Verification items for the finished model (mm, model axes). A direction names the side the tool comes from. Coordinates: 2 decimals unless noted, no trailing zeros. Write each loop counter-clockwise with the first axis right and the second up, starting at its lowest first coordinate (ties: lowest second). Pieces come first, ordered by that corner, then holes. Notation, with made-up numbers: (29.5, -21.5) -> (34.5, -21.5) arc R21 ccw to (34.5, 12.5) -> close; hole circle Ø11 at (24, -29). An arc over 180 degrees is marked (long way). Write each question's results on one line, items separated by ' | '. Start each with the question number.
from build123d import *

# Parameters (mm, degrees)
SKETCH1_R                = 21.082
SKETCH1_R_2              = 17.526
BOSS_EXTRUDE1_DEPTH      = 196.85
BOSS_EXTRUDE1_DEPTH_BACK = 196.85
SKETCH2_R                = 3.175
CUT_EXTRUDE1_DEPTH       = 22.082


with BuildPart() as part:
    # Sketch1 → Boss-Extrude1 (new body, two sides)
    with BuildSketch(Plane(origin=(0, 0, 0), x_dir=(0, 0, -1), z_dir=(1, 0, 0))) as boss_extrude1_sk:
        Circle(SKETCH1_R)
        Circle(SKETCH1_R_2, mode=Mode.SUBTRACT)
    extrude(amount=BOSS_EXTRUDE1_DEPTH)
    extrude(boss_extrude1_sk.sketch, amount=-BOSS_EXTRUDE1_DEPTH_BACK)

    # Sketch2 → Cut-Extrude1 (cut, through all)
    with BuildSketch(Plane.XY):
        with Locations((-114.3, 0)):
            Circle(SKETCH2_R)
        with Locations((-165.1, 0)):
            Circle(SKETCH2_R)
    extrude(amount=CUT_EXTRUDE1_DEPTH, mode=Mode.SUBTRACT)


solid = part.part
1. Sectioned sample at B-B on y = -14. Record the cut outline in (x, z).
2. Tool access check on faces 1 (the flat face through (196.85, 16, 8)), 2 (the cylindrical face through (-117.47, 0.14, 19.13)). Record the directions out of +Z, -Z, +X, -X, +Y, -Y that give a thin tool (end or side, any length) a straight path to the whole face; none if there is none.
3. Sectioned sample at A-A on z = 0. Record the cut outline in (x, y), plus the area to 3 significant figures.
4. Material ranges on probe 1 along Y at (x, z) = (-139, 0); probe 2 along Y at (x, z) = (-124, -9), recorded low to high. Write a range as from..to.
5. Sectioned sample at C-C on x = 141. Record the cut outline in (y, z).
6. Depth check by flat-ended pin: pin 1 Ø1 at (x, z) = (1.5, 7.5) entering from -Y; pin 2 Ø4 at (x, z) = (-119, -4) entering from -Y; pin 3 Ø5 at (x, y) = (-114.3, 0) entering from +Z. Enter the tip coordinate at first touch or a pass-through.
7. Mould release check, pull along Y, two halves, no side actions. Record for faces 3 (the flat face through (-196.85, 16, 8)), 4 (the cylindrical face through (-168.27, 0.14, 19.13)), 5 (the cylindrical face through (2.76, 6.33, -20.11)): +Y half, -Y half, draft (parallel to the pull), parting line (faces both ways), or undercut.
Computed values:
1) outline: (-196.85, -15.76) -> (196.85, -15.76) -> (196.85, -10.54) -> (-196.85, -10.54) -> close; (-196.85, 10.54) -> (196.85, 10.54) -> (196.85, 15.76) -> (-196.85, 15.76) -> close
2) face 1: +Z, -Z, +X, +Y, -Y | face 2: +Z
3) outline: (-196.85, -21.08) -> (196.85, -21.08) -> (196.85, -17.53) -> (-196.85, -17.53) -> close; (-196.85, 17.53) -> (196.85, 17.53) -> (196.85, 21.08) -> (-196.85, 21.08) -> close | area: 2,800 mm^2
4) probe 1: y = -21.08..-17.53, 17.53..21.08 | probe 2: y = -19.06..-15.04, 15.04..19.06
5) outline: circle Ø42.16 at (0, 0); hole circle Ø35.05 at (0, 0)
6) pin 1: stops at y = -19.89 | pin 2: stops at y = -20.99 | pin 3: stops at z = -17.35
7) face 3: draft | face 4: undercut | face 5: parting line
